Geometry check sheet. Reference: drawing and pictorial views, mm from the part's lowest x, y, z. A direction names the side the tool comes from. Round coordinates to 2 decimals unless told otherwise and drop trailing zeros. Loops run counter-clockwise (first coordinate to the right, second up) from the corner with the lowest first, then second, coordinate; pieces in that order, holes last. Notation, with made-up numbers: (47.25, 37) - (55.25, 37) arc R24 cw to (55.25, 74) - close; hole circle Ø5 at (-26, -24.5). An arc over 180 degrees is marked (long way). Return JSON: item names as keys, results as strings.
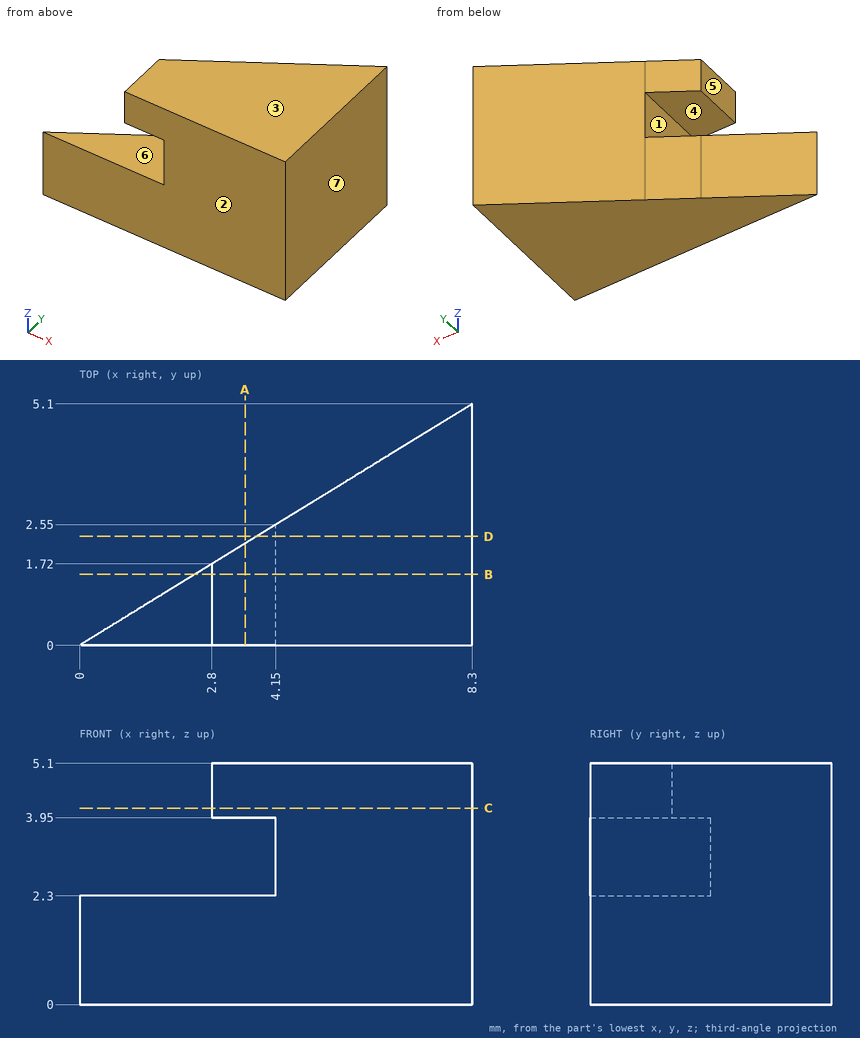
Q1. Depth check by flat-ended pin: P1, Ø0.8, axis at y = 1.5, z = 3, coming from the -X side; P2, Ø0.9, axis at y = 0.5, z = 5, coming from the -X side. Enter the tip coordinate at first touch or a pass-through.
Answer key:
{"P1": "stops at x = 4.15", "P2": "stops at x = 2.8"}
Q2. Scan lines: probe 1 along X at (y, z) = (0.4, 2.95); probe 2 along Y at (x, z) = (6.75, 3.75); probe 3 along Z at (x, y) = (2.75, 0.3). Record each from-to range of solid material in increasing order. Write a range as [from, to].
Answer key:
{"probe 1": "x = [4.15, 8.3]", "probe 2": "y = [0, 4.15]", "probe 3": "z = [0, 2.3]"}
Q3. Tool access check on the marked faces 5, 6 and 7. Record the directions out of +Z, -Z, +X, -X, +Y, -Y that give a thin tool (end or side, any length) a straight path to the whole face; none if there is none.
Answer key:
{"face 5": "+Z, -X, +Y, -Y", "face 6": "-X, +Y, -Y", "face 7": "+Z, -Z, +X, +Y, -Y"}
Q4. Sectioned sample at A-A (x = 3.5). Enter the section's corners in (y, z).
Answer key:
{"outline": "(0, 0) - (2.15, 0) - (2.15, 2.3) - (0, 2.3) - close; (0, 3.95) - (2.15, 3.95) - (2.15, 5.1) - (0, 5.1) - close"}
Q5. Draft check along Z on the marked faces 1, 2, 3 and 4. Enter one of: released by +Z, released by -Z, zero draft, split by the parting line, or undercut.
Answer key:
{"face 1": "undercut", "face 2": "zero draft", "face 3": "released by +Z", "face 4": "undercut"}
Q6. Sectioned sample at C-C (z = 4.15). Enter the section's corners in (x, y).
Answer key:
{"outline": "(2.8, 0) - (8.3, 0) - (8.3, 5.1) - (2.8, 1.72) - close"}
Q7. Sectioned sample at B-B (y = 1.5). Enter the section's corners in (x, z).
Answer key:
{"outline": "(2.44, 0) - (8.3, 0) - (8.3, 5.1) - (2.8, 5.1) - (2.8, 3.95) - (4.15, 3.95) - (4.15, 2.3) - (2.44, 2.3) - close"}
Q8. Sectioned sample at D-D (y = 2.3). Enter the section's corners in (x, z).
Answer key:
{"outline": "(3.74, 0) - (8.3, 0) - (8.3, 5.1) - (3.74, 5.1) - (3.74, 3.95) - (4.15, 3.95) - (4.15, 2.3) - (3.74, 2.3) - close"}
